The model under review builds one solid part; all positions refer to its coordinate system, in mm. Round coordinates to 2 decimals unless told otherwise and drop trailing zeros. Write each loop counter-clockwise with the first axis right and the second up, starting at its lowest first coordinate (ties: lowest second). Pieces come first, ordered by that corner, then holes. Notation, with made-up numbers: (78, -11.5) - (114, -11.5) arc R24 cw to (114, 16.5) - close; hole circle Ø4 at (14.25, 88). An arc over 180 degrees is marked (long way). Use one line per item in the form item = value.
Autodesk Fusion 360 part; units mm, degrees
sketch "Back Panel" plane through (0, 0, 0) normal (1, 0, 0) x (0, 1, 0)
  line L0 (0, 0) -> (6, 0)
  line L1 (6, 0) -> (6, 500.8)
  line L2 (0, 500.8) -> (0, 0)
  line L3 (0, 500.8) -> (0, 503.263)
  line L4 (6, 500.8) -> (0, 503.263)
  dimension "d8" = 6
  dimension "d9" = 500.8
  dimension "d10" = 2.463
  dimension "d11" = 112.318
extrude "Extrude2" add sketch "Back Panel" along normal blind 270
sketch "Switch Hole" plane through (0, 6, 0) normal (0, 1, 0) x (-1, 0, 0)
  line L0 (0, 0) -> (0, 500.8)
  line L1 (0, 500.8) -> (-270, 500.8)
  line L2 (-270, 500.8) -> (-270, 0)
  line L3 (-270, 0) -> (0, 0)
  line L4 (-234, 36) -> (-216, 36)
  line L5 (-216, 36) -> (-216, 24)
  line L6 (-216, 24) -> (-234, 24)
  line L7 (-234, 24) -> (-234, 36)
  dimension "d14" = 18
  dimension "d15" = 12
  dimension "d16" = 36
  dimension "d17" = 24
extrude "Extrude3" cut sketch "Switch Hole" against normal blind 6 contours L4 L5 L6 L7
sketch "Bottom Access Panel" plane through (0, 6, 0) normal (0, 1, 0) x (-1, 0, 0)
  line L0 (-216, 36) -> (-216, 24)
  line L1 (-216, 24) -> (-234, 24)
  line L2 (-234, 24) -> (-234, 36)
  line L3 (-234, 36) -> (-216, 36)
  line L4 (0, 0) -> (0, 500.8)
  line L5 (0, 500.8) -> (-270, 500.8)
  line L6 (-270, 500.8) -> (-270, 0)
  line L7 (-270, 0) -> (0, 0)
  line L8 (-205, 188) -> (-65, 188)
  line L9 (-65, 188) -> (-65, 48)
  line L10 (-65, 48) -> (-205, 48)
  line L11 (-205, 48) -> (-205, 188)
  dimension "d20" = 48
  dimension "d21" = 65
  dimension "d22" = 65
  dimension "d28" = 140
  dimension "d29" = 140
  dimension "d30" = 24
  dimension "d31" = 12
  dimension "d32" = 12
  dimension "d33" = 188
extrude "Extrude4" cut sketch "Bottom Access Panel" against normal blind 6 contours L8 L9 L10 L11
fillet "Fillet1" radius 8 4 edges at (65, 3, 188) (65, 3, 48) (205, 3, 48) (205, 3, 188)
sketch "Top Access Panel" plane through (0, 6, 0) normal (0, 1, 0) x (-1, 0, 0)
  line L0 (-65, 180) -> (-65, 56)
  arc A0 (-73, 48) -> (-65, 56) centre (-73, 56) ccw
  line L1 (-73, 48) -> (-197, 48)
  arc A1 (-205, 56) -> (-197, 48) centre (-197, 56) ccw
  line L2 (-205, 56) -> (-205, 180)
  arc A2 (-197, 188) -> (-205, 180) centre (-197, 180) ccw
  line L3 (-197, 188) -> (-73, 188)
  arc A3 (-65, 180) -> (-73, 188) centre (-73, 180) ccw
  line L4 (-216, 36) -> (-216, 24)
  line L5 (-216, 24) -> (-234, 24)
  line L6 (-234, 24) -> (-234, 36)
  line L7 (-234, 36) -> (-216, 36)
  line L8 (0, 0) -> (0, 500.8)
  line L9 (0, 500.8) -> (-270, 500.8)
  line L10 (-270, 500.8) -> (-270, 0)
  line L11 (-270, 0) -> (0, 0)
  line L12 (-195, 473.263) -> (-75, 473.263)
  line L13 (-75, 473.263) -> (-75, 383.263)
  line L14 (-75, 383.263) -> (-195, 383.263)
  line L15 (-195, 383.263) -> (-195, 473.263)
  line L16 (-180, 473.263) -> (-90, 473.263)
  line L17 (0, 503.263) -> (-270, 503.263)
  dimension "d34" = 120
  dimension "d35" = 140
  dimension "d36" = 75
  dimension "d37" = 75
  dimension "d38" = 65
  dimension "d39" = 65
  dimension "d45" = 90
  dimension "d49" = 30
extrude "Extrude5" cut sketch "Top Access Panel" against normal blind 6 contours L12 L13 L14 L15 L16
fillet "Fillet2" radius 8 4 edges at (75, 3, 473.263) (195, 3, 473.263) (195, 3, 383.263) (75, 3, 383.263)
equation "MDFThickness = 6 mm"
equation "d16 = ( 18 * 2 ) * 1 mm"
equation "d17 = ( 12 * 2 ) * 1 mm"
equation "filletRadius = 8 mm"
equation "d27 = filletRadius"
equation "d36 = ( ( 270 - 120 ) / 2 ) * 1 mm"
equation "d54 = filletRadius"
(1) Add section D-D on z = 457.5. Write out the cut boundary in (x, y), then the cut area to 3 significant figures.
Geometry results:
outline = (0, 0) - (75, 0) - (75, 6) - (0, 6) - close; (195, 0) - (270, 0) - (270, 6) - (195, 6) - close
area = 900 mm2
(2) Add section C-C on y = 4.6. Write out the cut boundary in (x, z), then the cut area to 3 significant figures.
Geometry results:
outline = (0, 0) - (270, 0) - (270, 501.37) - (0, 501.37) - close; hole (65, 56) arc R8 ccw to (73, 48) - (197, 48) arc R8 ccw to (205, 56) - (205, 180) arc R8 ccw to (197, 188) - (73, 188) arc R8 ccw to (65, 180) - close; hole (75, 391.26) arc R8 ccw to (83, 383.26) - (187, 383.26) arc R8 ccw to (195, 391.26) - (195, 465.26) arc R8 ccw to (187, 473.26) - (83, 473.26) arc R8 ccw to (75, 465.26) - close; hole (216, 24) - (234, 24) - (234, 36) - (216, 36) - close
area = 105,000 mm2
(3) Add section B-B on x = 97. Write out the cut boundary in (y, z).
Geometry results:
outline = (0, 0) - (6, 0) - (6, 48) - (0, 48) - close; (0, 188) - (6, 188) - (6, 383.26) - (0, 383.26) - close; (0, 473.26) - (6, 473.26) - (6, 500.8) - (0, 503.26) - close
(4) To check wall thickness, follow L1, parallel to X at y = 2.15, z = 448; L2, parallel to X at y = 4.1, z = 113; L3, parallel to Z at x = 123, y = 5.45. State the ranges of each line that lie inside material, in increasing order.
Geometry results:
L1 = 0 to 75, 195 to 270
L2 = 0 to 65, 205 to 270
L3 = 0 to 48, 188 to 383.26, 473.26 to 501.03
(5) Add section A-A on z = 151.5. Write out the cut boundary in (x, y).
Geometry results:
outline = (0, 0) - (65, 0) - (65, 6) - (0, 6) - close; (205, 0) - (270, 0) - (270, 6) - (205, 6) - close
(6) Insertion check: P1, Ø3, axis at x = 228, y = 4, coming from the +Z side; P2, Ø1.8, axis at x = 127.5, y = 2.5, coming from the +Z side. Each pin has a flat end and moves straight along its axis. Give the tip position at first contact, or say it passes through.
Geometry results:
P1 = 502.24
P2 = 502.61
